Read the model definition and answer for the solid it produces. Units are mm, in the model's axes. Give positions to 0.01 mm unless a question says otherwise; leave off trailing zeros. Loops run counter-clockwise (first coordinate to the right, second up) from the corner with the lowest first, then second, coordinate; pieces in that order, holes last. Notation, with made-up numbers: (82.25, 37) - (88.25, 37) arc R36 cw to (88.25, 74) - close; hole circle Ø1 at (86.5, 15.5). An arc over 180 degrees is marked (long way). Write item = value, one per line.
```python
from build123d import *

# Parameters (mm, degrees)
BOSS_EXTRUDE1_DEPTH = 38.1
SKETCH3_R           = 3.175
CUT_EXTRUDE1_DEPTH  = 38.1


with BuildPart() as part:
    # Sketch2 → Boss-Extrude1 (new body)
    with BuildSketch(Plane(origin=(0, 0, 0), x_dir=(1, 0, 0), z_dir=(0, 1, 0))):
        with BuildLine():
            ThreePointArc((-79.131998656, -36.899856978), (-85.242845122, -18.897883792), (-87.3125, 0))
            Line((-87.3125, 0), (-88.9, 0))
            ThreePointArc((-88.9, 0), (-86.792715033, -19.241481679), (-80.570762268, -37.570763469))
            Line((-80.570762268, -37.570763469), (-79.131998656, -36.899856978))
        make_face()
    extrude(amount=BOSS_EXTRUDE1_DEPTH)

    # Sketch3 → Cut-Extrude1 (cut)
    with BuildSketch(Plane(origin=(-86.792715033, 0, 19.241481679), x_dir=(0, -1, 0), z_dir=(-0.976296007, 0, 0.216439614))):
        with Locations((-31.75, -12.7)):
            Circle(SKETCH3_R)
        with Locations((-31.75, 12.7)):
            Circle(SKETCH3_R)
        with Locations((-6.35, -12.7)):
            Circle(SKETCH3_R)
        with Locations((-6.35, 12.7)):
            Circle(SKETCH3_R)
    extrude(amount=-CUT_EXTRUDE1_DEPTH, mode=Mode.SUBTRACT)


solid = part.part
```
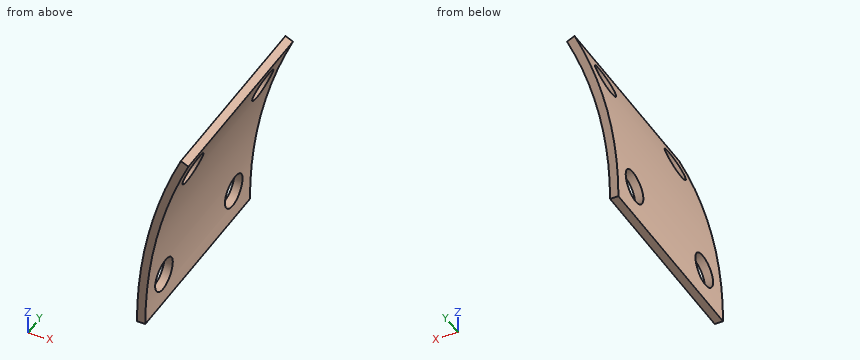
1) Find the intervals of material crossed by probe 1 along X at (y, z) = (11, 8); probe 2 along X at (y, z) = (15, 33.5); probe 3 along Z at (x, y) = (-81, 35.5), in increasing order.
Output:
probe_1 = -88.54 to -86.95
probe_2 = -82.35 to -80.63
probe_3 = 32.6 to 36.64
2) A cutting plane is placed at B-B on z = 4.5. Give the number of separate pieces and of enclosed holes in the cut face, then the cut area to 3 significant figures.
Output:
separate_pieces = 3
enclosed_holes = 0
area = 44.7 mm²
3) A cutting plane is placed at C-C on z = 25. Determine the outline of the cut face in (x, y).
Output:
outline = (-85.31, 0) - (-83.66, 0) - (-83.66, 38.1) - (-85.31, 38.1) - close
4) Each of these flat-tipped pins is pushed along its axis until it touches: P1, Ø2, axis at x = -82.5, y = 4, coming from the +Z side; P2, Ø4, axis at x = -86, y = 32, coming from the +Z side; P3, Ø12, axis at y = 32.5, z = 15, coming from the -X side. Where does it stop, or does it pass through?
Output:
P1 = 35.51
P2 = 28.6
P3 = -88.43
5) A cutting plane is placed at A-A on y = 24. Determine the outline of the cut face in (x, z) (1 decimal), then the cut area to 3 significant figures.
Output:
outline = (-88.9, 0) - (-87.3, 0) arc R87.3 cw to (-79.1, 36.9) - (-80.6, 37.6) arc R88.9 ccw to start
area = 61.0 mm²
